Job drawing, mm, ordinate dimensions from the low corner. One solid piece. Round coordinates to 2 decimals unless told otherwise and drop trailing zeros. Loops run counter-clockwise (first coordinate to the right, second up) from the corner with the lowest first, then second, coordinate; pieces in that order, holes last.
1) Drop a flat-ended pin along its axis: P1, Ø2.5, axis at x = 10, z = 32.5, coming from the +Y side. Give the stop position or say it passes through.
2) Band-saw the part on A-A, the plane x = 140. Write the cut outline in (y, z).
3) Probe line 1 (X direction, y = 1, z = 20.5); line 2 (Z direction, x = 75, y = 0.9); line 3 (X direction, y = 0.6, z = 32.5). List the from-to ranges inside material, lowest first.
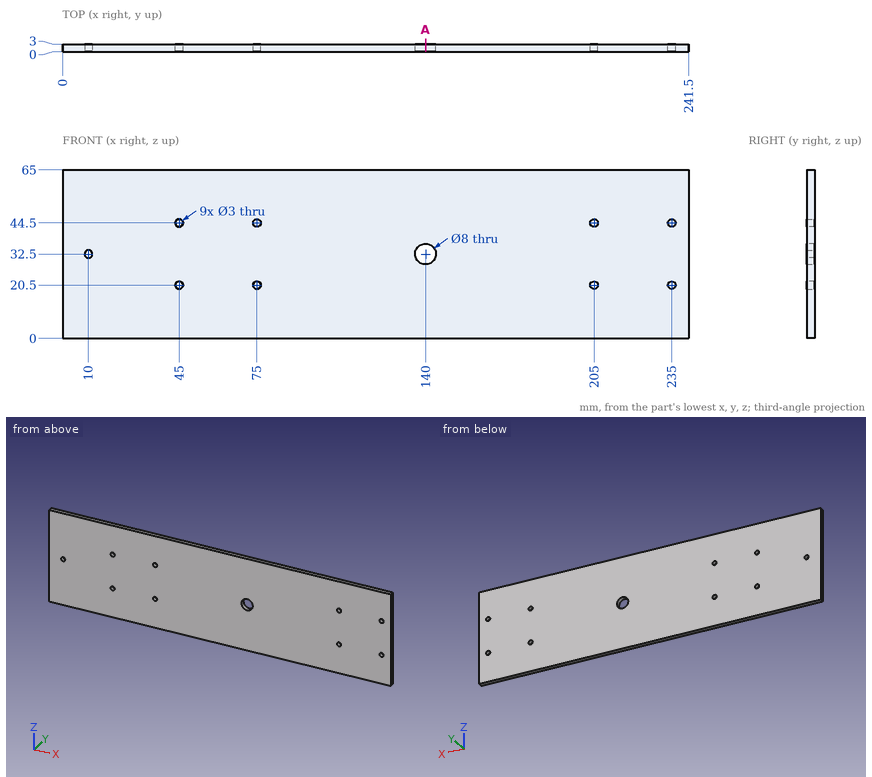
Reported:
1. P1: passes through
2. outline: (0, 0) - (3, 0) - (3, 28.5) - (0, 28.5) - close; (0, 36.5) - (3, 36.5) - (3, 65) - (0, 65) - close
3. line 1: x = 0 to 43.5, 46.5 to 73.5, 76.5 to 203.5, 206.5 to 233.5, 236.5 to 241.5
3. line 2: z = 0 to 19, 22 to 43, 46 to 65
3. line 3: x = 0 to 8.5, 11.5 to 136, 144 to 241.5
